Part model, mm, in its own coordinate system. Face numbers are marked on the shaded views. A direction names the side the tool comes from. Coordinates: 2 decimals unless noted, no trailing zeros. Write each loop counter-clockwise with the first axis right and the second up, starting at its lowest first coordinate (ties: lowest second). Pieces come first, ordered by that corner, then holes. Notation, with made-up numbers: (48.5, -14) -> (54.5, -14) arc R24 cw to (54.5, 13) -> close; hole circle Ø11 at (-8.5, 65.25). An arc over 180 degrees is marked (long way). Write item = value, one per line.
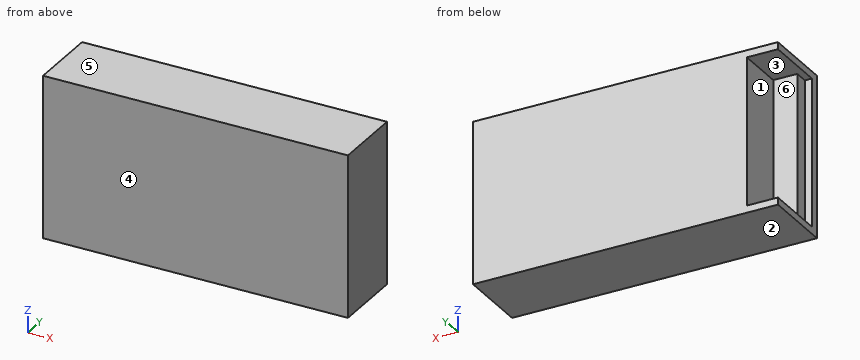
from build123d import *

# Parameters (mm, degrees)
ESBO_O1_W                = 215
ESBO_O1_H                = 114
RESSALTO_EXTRUS_O1_DEPTH = 50
CORTE_EXTRUS_O1_START    = -109
CORTE_EXTRUS_O1_DEPTH    = 104


with BuildPart() as part:
    # Esboço1 → Ressalto-extrusão1 (new body)
    with BuildSketch(Plane(origin=(0, 0, 0), x_dir=(1, 0, 0), z_dir=(0, 1, 0))):
        Rectangle(ESBO_O1_W, ESBO_O1_H)
    extrude(amount=RESSALTO_EXTRUS_O1_DEPTH)

    # Esboço3 → Corte-extrusão1 (cut)
    with BuildSketch(Plane.XY.offset(57).offset(CORTE_EXTRUS_O1_START)):
        Polygon((-107.5, 50), (-85.58523496, 50), (-85.58523496, 16.13389081), (-102.483117777, 16.13389081), (-102.483117777, 6.426889092), (-107.5, 6.426889092), (-107.5, 17.457061978), align=None)
    extrude(amount=CORTE_EXTRUS_O1_DEPTH, mode=Mode.SUBTRACT)


solid = part.part
Q1. Mould opens along Z. For the marked faces 1, 2, 3 and 4 say: released by +Z, released by -Z, zero draft, split by the parting line, or undercut.
Model answer:
face_1 = undercut
face_2 = released by -Z
face_3 = undercut
face_4 = zero draft
Q2. Saw through at A-A on y = 10.5. Give the cut face in (x, z), and give its area (3 significant figures).
Model answer:
outline = (-107.5, -57) -> (107.5, -57) -> (107.5, 57) -> (-107.5, 57) -> (-107.5, 52) -> (-102.48, 52) -> (-102.48, -52) -> (-107.5, -52) -> close
area = 24,000 mm²
Q3. Saw through at B-B on z = -2. Give the cut face in (x, y).
Model answer:
outline = (-107.5, 0) -> (107.5, 0) -> (107.5, 50) -> (-85.59, 50) -> (-85.59, 16.13) -> (-102.48, 16.13) -> (-102.48, 6.43) -> (-107.5, 6.43) -> close
Q4. Probe line 1 (X direction, y = 20.5, z = -1); line 2 (X direction, y = 12.5, z = 23); line 3 (Z direction, x = -87, y = 41.5). List the from-to ranges inside material, lowest first. Write a range as from..to.
Model answer:
line_1 = -85.59..107.5
line_2 = -102.48..107.5
line_3 = -57..-52, 52..57
Q5. Pin check, flat tips, straight feed: pin 1 (8 mm diameter, centred on y = 10.5, z = -19, fed in from -X); pin 2 (1.5 mm diameter, centred on x = -34, z = -8, fed in from -Y); pin 3 (2.5 mm diameter, centred on x = -105.5, z = -20.5, fed in from +Y); pin 4 (3 mm diameter, centred on y = 37.5, z = -6.5, fed in from -X). Stop position of each tip, or through.
Model answer:
pin_1 = -102.48
pin_2 = 0
pin_3 = 6.43
pin_4 = -85.59
Q6. Which spindle directions (+Z, -Z, +X, -X, +Y, -Y) get a long thin tool onto all of the face, cutting with end or side? Do the marked faces 5 and 6. Say none if no direction does.
Model answer:
face_5 = +Z, +X, -X, +Y, -Y
face_6 = -X, +Y
